```python
from build123d import *

# Parameters (mm, degrees)
CROQUIS1_R              = 22.5
CROQUIS1_R_2            = 18.25
SALIENTE_EXTRUIR1_DEPTH = 30
SALIENTE_EXTRUIR2_DEPTH = 11.6
SALIENTE_EXTRUIR3_DEPTH = 11.6


with BuildPart() as part:
    # Croquis1 → Saliente-Extruir1 (new body)
    with BuildSketch(Plane.XY):
        Circle(CROQUIS1_R)
        Circle(CROQUIS1_R_2, mode=Mode.SUBTRACT)
    extrude(amount=SALIENTE_EXTRUIR1_DEPTH)

    # Croquis2 → Saliente-Extruir2 (add)
    with BuildSketch(Plane.XY.offset(30)):
        with BuildLine():
            Line((-18.708286934, 12.5), (18.708286934, 12.5))
            ThreePointArc((18.708286934, 12.5), (0, 22.5), (-18.708286934, 12.5))
        make_face()
        with BuildLine():
            Line((-18.708286934, -12.5), (18.708286934, -12.5))
            ThreePointArc((18.708286934, -12.5), (0, -22.5), (-18.708286934, -12.5))
        make_face()
    extrude(amount=SALIENTE_EXTRUIR2_DEPTH)

    # Croquis3 → Saliente-Extruir3 (add)
    with BuildSketch(Plane.XY.offset(30)):
        with BuildLine():
            Line((18.708286934, 12.5), (13.297086147, 12.5))
            ThreePointArc((13.297086147, 12.5), (18.25, 0), (13.297086147, -12.5))
            Line((13.297086147, -12.5), (18.708286934, -12.5))
            ThreePointArc((18.708286934, -12.5), (22.5, 0), (18.708286934, 12.5))
        make_face()
        with BuildLine():
            Line((-13.297086147, 12.5), (-18.708286934, 12.5))
            ThreePointArc((-18.708286934, 12.5), (-22.5, 0), (-18.708286934, -12.5))
            Line((-18.708286934, -12.5), (-13.297086147, -12.5))
            ThreePointArc((-13.297086147, -12.5), (-18.25, 0), (-13.297086147, 12.5))
        make_face()
    extrude(amount=SALIENTE_EXTRUIR3_DEPTH)


solid = part.part
```
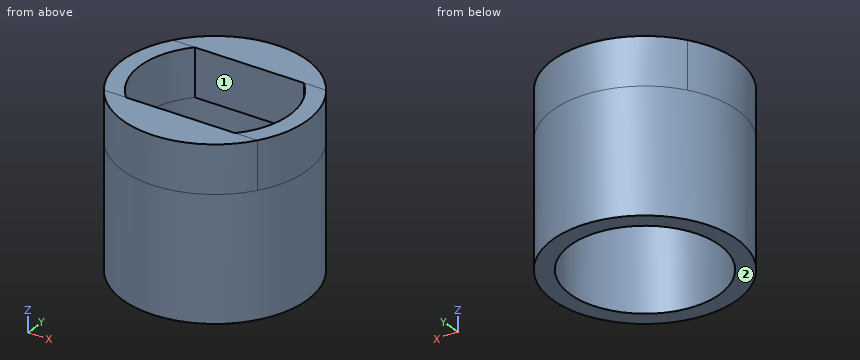
Here's how the part is built. I have some questions about the finished solid (model axes, mm). Face numbers are marked on the shaded views. Give positions to 0.01 mm unless a question says otherwise; leave off trailing zeros. Order: outer loops, then holes, each group sorted by start corner. A loop starts at its lowest first (then second) coordinate and runs counter-clockwise, first axis right, second up. Notation, with made-up numbers: M 74.5,-18 L 102.5,-18 A10 ccw 102.5,-8 Z; hole C -26,45.5 d5. An arc over 180 degrees is marked long. Use a Markdown table: item, result. Add a question column.
1. I need wall thicknesses on probe 1 along Y at (x, z) = (0, 20); probe 2 along Z at (x, y) = (-4, 13.5); probe 3 along Y at (x, z) = (0.5, 34.5). Which ranges of each line are inside material? Lowest first, please. Write a range as from..to.
2. Suppose I cut it at D-D (y = 9). List the corners of the cut face in (x, z) for me, and give its area (3 significant figures).
3. If we mould it in two halves opening along X, with no side actions, what happens to the marked faces 1 and 2? For each: +X half, -X half, draft (parallel to the pull), parting line (faces both ways), or undercut.
4. For pin 1 Ø5 at (x, z) = (8, 15.5) entering from +Y; pin 2 Ø13 at (x, z) = (-2, 38) entering from -Y; pin 3 Ø12 at (x, z) = (-11, 17) entering from +Y; pin 4 Ø3 at (x, y) = (5.5, 14) entering from -Z, each with a flat end and sliding along its axis, tell me the tip position at first contact or that it passes through.
5. Suppose I cut it at A-A (y = 0). List the corners of the cut face in (x, z) for me.
6. Suppose I cut it at B-B (z = 38). List the corners of the cut face in (x, y) for me.
7. Suppose I cut it at C-C (x = 0). List the corners of the cut face in (y, z) for me.
Results list:
| question | item | result |
|---|---|---|
| 1 | probe 1 | y = -22.5..-18.25, 18.25..22.5 |
| 1 | probe 2 | z = 30..41.6 |
| 1 | probe 3 | y = -22.49..-12.5, 12.5..22.49 |
| 2 | outline | M -20.62,0 L -15.88,0 L -15.88,41.6 L -20.62,41.6 Z; M 15.88,0 L 20.62,0 L 20.62,41.6 L 15.88,41.6 Z |
| 2 | area | 395 mm² |
| 3 | face 1 | undercut |
| 3 | face 2 | draft |
| 4 | pin 1 | stops at y = 21.82 |
| 4 | pin 2 | stops at y = -22.5 |
| 4 | pin 3 | stops at y = 21.94 |
| 4 | pin 4 | stops at z = 30 |
| 5 | outline | M -22.5,0 L -18.25,0 L -18.25,41.6 L -22.5,41.6 Z; M 18.25,0 L 22.5,0 L 22.5,41.6 L 18.25,41.6 Z |
| 6 | outline | C 0,0 d45; hole M -13.3,-12.5 L 13.3,-12.5 A18.25 ccw 13.3,12.5 L -13.3,12.5 A18.25 ccw Z |
| 7 | outline | M -22.5,0 L -18.25,0 L -18.25,30 L -12.5,30 L -12.5,41.6 L -22.5,41.6 Z; M 12.5,30 L 18.25,30 L 18.25,0 L 22.5,0 L 22.5,41.6 L 12.5,41.6 Z |
